from build123d import *

# Parameters (mm, degrees)
BOSS_EXTRUDE1_DEPTH         = 9.525
M5_CLEARANCE_HOLE1_D        = 5.5
M5_CLEARANCE_HOLE1_DEPTH    = 18.75
M5_CLEARANCE_HOLE1_TIP      = 1.652366702
FILLET1_R                   = 3.175
F_1_4_CLEARANCE_HOLE1_D     = 6.7564
F_1_4_CLEARANCE_HOLE1_DEPTH = 18.75
F_1_4_CLEARANCE_HOLE1_TIP   = 2.029827343
SKETCH7_W                   = 70.609127035
SKETCH7_H                   = 15.5
CUT_EXTRUDE1_DEPTH          = 199.318467163
FILLET2_R                   = 3.175
SKETCH8_W                   = 20
SKETCH8_H                   = 61.78174593
BOSS_EXTRUDE2_DEPTH         = 9.525
FILLET3_R                   = 3.175


with BuildPart() as part:
    # Sketch1 → Boss-Extrude1 (new body)
    with BuildSketch(Plane.XY):
        Polygon((82.55, 31.75), (82.55, 50.890872965), (191.440872965, 50.890872965), (191.440872965, 30.890872965), (109.659127035, 30.890872965), (109.659127035, -30.890872965), (191.440872965, -30.890872965), (191.440872965, -50.890872965), (82.55, -50.890872965), (82.55, -31.75), (-31.75, -31.75), (-31.75, 31.75), align=None)
    extrude(amount=BOSS_EXTRUDE1_DEPTH)

    # M5 Clearance Hole1
    with Locations(Plane.XY.offset(9.525)):
        with Locations((179.440872965, 38.890872965), (179.440872965, -38.890872965), (101.659127035, 38.890872965), (101.659127035, -38.890872965)):
            Hole(M5_CLEARANCE_HOLE1_D / 2, depth=M5_CLEARANCE_HOLE1_DEPTH)
            with Locations((0, 0, -(M5_CLEARANCE_HOLE1_DEPTH + M5_CLEARANCE_HOLE1_TIP / 2))):  # 118° drill point
                Cone(0, M5_CLEARANCE_HOLE1_D / 2, M5_CLEARANCE_HOLE1_TIP, mode=Mode.SUBTRACT)

    # Fillet1
    fillet1_edges = [part.edges().sort_by_distance(p)[0] for p in [
        (82.55, 31.75, 4.7625),
        (109.659127035, 30.890872965, 4.7625),
        (109.659127035, -30.890872965, 4.7625),
        (82.55, -31.75, 4.7625),
    ]]
    fillet(fillet1_edges, radius=FILLET1_R)

    # 1/4 Clearance Hole1
    with Locations(Plane.XY.offset(9.525)):
        with Locations((-19.05, 19.05), (6.35, 19.05), (6.35, -19.05), (-19.05, -19.05)):
            Hole(F_1_4_CLEARANCE_HOLE1_D / 2, depth=F_1_4_CLEARANCE_HOLE1_DEPTH)
            with Locations((0, 0, -(F_1_4_CLEARANCE_HOLE1_DEPTH + F_1_4_CLEARANCE_HOLE1_TIP / 2))):  # 118° drill point
                Cone(0, F_1_4_CLEARANCE_HOLE1_D / 2, F_1_4_CLEARANCE_HOLE1_TIP, mode=Mode.SUBTRACT)

    # Sketch7 → Cut-Extrude1 (cut, through all)
    with BuildSketch(Plane.XY.offset(9.525)):
        with Locations((54.354563518, 0)):
            Rectangle(SKETCH7_W, SKETCH7_H)
    extrude(amount=-CUT_EXTRUDE1_DEPTH, mode=Mode.SUBTRACT)

    # Fillet2
    fillet2_edges = [part.edges().sort_by_distance(p)[0] for p in [
        (19.05, -7.75, 4.7625),
        (19.05, 7.75, 4.7625),
        (89.659127035, 7.75, 4.7625),
        (89.659127035, -7.75, 4.7625),
    ]]
    fillet(fillet2_edges, radius=FILLET2_R)

    # Sketch8 → Boss-Extrude2 (add)
    with BuildSketch(Plane.XY.offset(9.525)):
        with Locations((181.440872965, 0)):
            Rectangle(SKETCH8_W, SKETCH8_H)
    extrude(amount=-BOSS_EXTRUDE2_DEPTH)

    # Fillet3
    fillet3_edges = [part.edges().sort_by_distance(p)[0] for p in [
        (171.440872965, 30.890872965, 4.7625),
        (171.440872965, -30.890872965, 4.7625),
    ]]
    fillet(fillet3_edges, radius=FILLET3_R)


solid = part.part
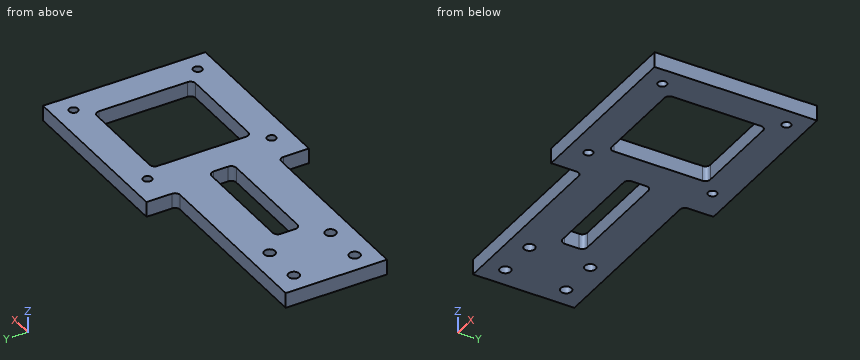
The model under review builds one solid part; all positions refer to its coordinate system, in mm. Give positions to 0.01 mm unless a question says otherwise; leave off trailing zeros. Write each loop counter-clockwise with the first axis right and the second up, starting at its lowest first coordinate (ties: lowest second). Pieces come first, ordered by that corner, then holes. Notation, with made-up numbers: M 55,-37.75 L 102,-37.75 A17 ccw 102,-5.75 Z; hole C -7.5,40.25 d2. An arc over 180 degrees is marked long. One line per question, with ' | ' between items. Start each with the question number.
Item 1: We need section D-D on z = 8. Give the number of separate pieces and of enclosed holes in the cut face, plus the area to 3 significant figures.
Item 2: We need section B-B on x = 126. Write out the cut boundary in (y, z) (3 decimals).
Item 3: We need section C-C on x = -19.05. Write out the cut boundary in (y, z) (3 decimals), plus the area to 3 significant figures.
Item 4: We need section A-A on y = -19.05. Write out the cut boundary in (x, z) (3 decimals).
Item 5: For pin 1 (1.5 mm diameter, centred on x = 79.5, z = 8, fed in from -Y); pin 2 (6 mm diameter, centred on x = -19.05, y = -19.05, fed in from +Z); pin 3 (5 mm diameter, centred on y = -39.5, z = 1.5, fed in from -X), all flat-tipped, find the tip position at first contact; note any pin that passes through.
Item 6: Wall thickness on line 1 (Y direction, x = 6.35, z = 5.25); line 2 (X direction, y = 37, z = 8); line 3 (X direction, y = 3.5, z = 7): over which ranges is each line inside the solid? List them lowest first. Write a range as from..to.
Results found:
1) separate pieces: 1 | enclosed holes: 10 | area: 13,200 mm2
2) outline: M -50.891,0 L -30.891,0 L -30.891,9.525 L -50.891,9.525 Z; M 30.891,0 L 50.891,0 L 50.891,9.525 L 30.891,9.525 Z
3) outline: M -31.75,0 L -22.428,0 L -22.428,9.525 L -31.75,9.525 Z; M -15.672,0 L 15.672,0 L 15.672,9.525 L -15.672,9.525 Z; M 22.428,0 L 31.75,0 L 31.75,9.525 L 22.428,9.525 Z | area: 476 mm2
4) outline: M -31.75,0 L -22.428,0 L -22.428,9.525 L -31.75,9.525 Z; M -15.672,0 L 2.972,0 L 2.972,9.525 L -15.672,9.525 Z; M 9.728,0 L 109.659,0 L 109.659,9.525 L 9.728,9.525 Z; M 171.441,0 L 191.441,0 L 191.441,9.525 L 171.441,9.525 Z
5) pin 1: stops at y = -31.87 | pin 2: passes through | pin 3: stops at x = 82.55
6) line 1: y = -31.75..-22.43, -15.67..15.67, 22.43..31.75 | line 2: x = 82.55..99.66, 103.66..177.44, 181.44..191.44 | line 3: x = -31.75..19.05, 89.66..109.66, 171.44..191.44
